from build123d import *

# Parameters (mm, degrees)
F1_DEPTH = 129
F3_DEPTH = 25
F5_DEPTH = 40
F8_DEPTH = 4


# Not quite as in the source:
# - a feature names something its author has since deleted; it is built from what else it names


with BuildPart() as f1:
    # F0 (on Right) → F1 (new body)
    with BuildSketch(Plane.YZ):
        with BuildLine():
            Line((12.6334434892, 34.7101007166), (0, 0))
            Line((0, 0), (3, 0))
            Line((3, 0), (15.7389581993, 35))
            Line((15.7389581993, 35), (30.7389581993, 35))
            Line((30.7389581993, 35), (30.7389581993, 38))
            Line((30.7389581993, 38), (17.3319065932, 38))
            ThreePointArc((17.3319065932, 38), (14.4640244114, 37.0957602214), (12.6334434892, 34.7101007166))
        make_face()
    extrude(amount=F1_DEPTH)

    # F2 (on face) → F3 (cut)
    with BuildSketch(Plane(origin=(0, 0, 0), x_dir=(1, 0, 0), z_dir=(0, -0.9396926208, 0.3420201433))):
        with BuildLine():
            Line((24.75, 7), (110.25, 7))
            ThreePointArc((110.25, 7), (111.6642135624, 7.5857864376), (112.25, 9))
            Line((112.25, 9), (112.25, 29))
            ThreePointArc((112.25, 29), (111.6642135624, 30.4142135624), (110.25, 31))
            Line((110.25, 31), (24.75, 31))
            ThreePointArc((24.75, 31), (23.3357864376, 30.4142135624), (22.75, 29))
            Line((22.75, 29), (22.75, 9))
            ThreePointArc((22.75, 9), (23.3357864376, 7.5857864376), (24.75, 7))
        make_face()
        with BuildLine():
            ThreePointArc((-13.2679491924, 10), (-13.2679491924, 8), (-11.5358983849, 7))
            Line((-11.5358983849, 7), (0, 7))
            Line((0, 7), (0, 30.9807621135))
            ThreePointArc((0, 30.9807621135), (-1, 30.7128129211), (-1.7320508076, 29.9807621135))
            Line((-1.7320508076, 29.9807621135), (-13.2679491924, 10))
        make_face()
        with BuildLine():
            Line((0, 30.9807621135), (0, 7))
            Line((0, 7), (11.5358983849, 7))
            ThreePointArc((11.5358983849, 7), (13.2679491924, 8), (13.2679491924, 10))
            Line((13.2679491924, 10), (1.7320508076, 29.9807621135))
            ThreePointArc((1.7320508076, 29.9807621135), (1, 30.7128129211), (0, 30.9807621135))
        make_face()
    extrude(amount=-F3_DEPTH, mode=Mode.SUBTRACT)

    # F4 (on Front) → F5 (cut)
    with BuildSketch(Plane.XZ):
        Polygon((149, 50), (129, 50), (128, -10), (149, -10), align=None)
    extrude(amount=-F5_DEPTH, mode=Mode.SUBTRACT)

    # F7 (on offset) → F8 (join)
    with BuildSketch(Plane.YZ.offset(89)):
        Polygon((22.8702962437, 29.2118719039), (13.4733700358, 32.6320733372), (13.1313498925, 31.6923807164), (21.5885834796, 28.6141994265), (22.186255957, 27.3324866624), align=None)
    extrude(amount=F8_DEPTH)


solid = f1.part
The model under review builds one solid part; all positions refer to its coordinate system, in mm. A direction names the side the tool comes from. Coordinates: 2 decimals unless noted, no trailing zeros. Order: outer loops, then holes, each group sorted by start corner. A loop starts at its lowest first (then second) coordinate and runs counter-clockwise, first axis right, second up. Notation, with made-up numbers: (-18, 40.5) -> (1, 40.5) arc R17 ccw to (1, 71.5) -> close; hole circle Ø3 at (-14.75, -18.75). An arc over 180 degrees is marked (long way). Answer in a Markdown table with one row per item.
(1) Insertion check: pin 1 (2.5 mm diameter, centred on y = 18, z = 29.5, fed in from -X); pin 2 (7.5 mm diameter, centred on x = 33, y = 20, fed in from -Z); pin 3 (6 mm diameter, centred on x = 107.5, y = 7.5, fed in from +Z); pin 4 (1.5 mm diameter, centred on x = 94.5, y = 9.5, fed in from -Z). Each pin has a flat end and moves straight along its axis. Give the tip position at first contact, or say it passes through.
Answers:
| item | result |
|---|---|
| pin 1 | x = 89 |
| pin 2 | z = 35 |
| pin 3 | z = 5.81 |
| pin 4 | through |
(2) Consider section A-A (x = 44). Write out the cut boundary in (y, z).
Answers:
| item | result |
|---|---|
| outline | (0, 0) -> (3, 0) -> (5.04, 5.61) -> (2.39, 6.58) -> close; (10.6, 29.13) -> (13.25, 28.17) -> (15.74, 35) -> (30.74, 35) -> (30.74, 38) -> (17.33, 38) arc R5 ccw to (12.63, 34.71) -> close |
(3) Consider section D-D (y = 24). Write out the cut boundary in (x, z), plus the area to 3 significant figures.
Answers:
| item | result |
|---|---|
| outline | (0, 35) -> (128.75, 35) -> (128.8, 38) -> (0, 38) -> close |
| area | 386 mm² |
(4) Machinability: for faces 4 (the cylindrical face through (23.35, 11.71, 28.12)), 5 (the cylindrical face through (23.32, 3.906, 6.668)), 6 (the flat face through (89, 19, 30)), which of the approach directions +Z, -Z, +X, -X, +Y, -Y give a long, thin tool a straight path to every point of the face, cutting with its end or side? Answer none if there is none.
Answers:
| item | result |
|---|---|
| face 4 | -Z, -Y |
| face 5 | +Z, +Y |
| face 6 | -Z, -X, +Y |
(5) Consider section C-C (z = 18). Write out the cut boundary in (x, y), plus the area to 3 significant figures.
Answers:
| item | result |
|---|---|
| outline | (7.39, 9.55) -> (7.98, 6.55) -> (22.75, 6.55) -> (22.75, 9.55) -> close; (112.25, 6.55) -> (128.47, 6.55) -> (128.47, 9.55) -> (112.25, 9.55) -> close |
| area | 93.8 mm² |
(6) Wall thickness on line 1 along Z through (x, y) = (64, 25.5); line 2 along X through (y, z) = (24, 36.5) (3 decimals); line 3 along X through (y, z) = (8, 18): over which ranges is each line inside the solid? List them lowest first.
Answers:
| item | result |
|---|---|
| line 1 | 35 to 38 |
| line 2 | 0 to 128.775 |
| line 3 | 7.7 to 22.75, 112.25 to 128.47 |
(7) The part is to be moulded in two halves that separate along X. For faces 1 (the cylindrical face through (13.253, 4.034, 7.018)), 2 (the cylindrical face through (111.68, 11.7, 28.09)), 3 (the flat face through (63, 23, 35)), say which applies: +X half, -X half, draft (parallel to the pull), parting line (faces both ways), or undercut.
Answers:
| item | result |
|---|---|
| face 1 | -X half |
| face 2 | undercut |
| face 3 | draft |
(8) Consider section B-B (y = 19). Write out the cut boundary in (x, z).
Answers:
| item | result |
|---|---|
| outline | (0, 35) -> (128.75, 35) -> (128.8, 38) -> (0, 38) -> close; (89, 29.56) -> (93, 29.56) -> (93, 30.62) -> (89, 30.62) -> close |
